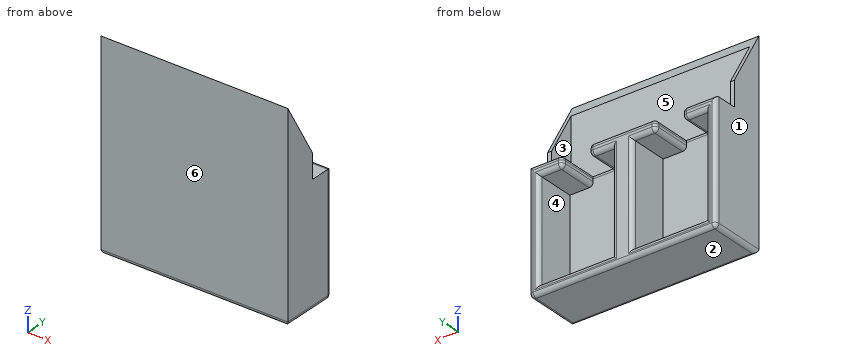
from build123d import *

# Parameters (mm, degrees)
SKETCH1_W               = 140
SKETCH1_H               = 90
BOSS_EXTRUDE1_DEPTH     = 42
CUT_EXTRUDE1_DEPTH      = 30
FILLET2_R               = 3
SKETCH3_W               = 140
SKETCH3_H               = 60
BOSS_EXTRUDE2_DEPTH     = 5
SKETCH4_W               = 3
SKETCH4_H               = 60
BOSS_EXTRUDE3_DEPTH     = 19
CUT_EXTRUDE2_DEPTH      = 172.650808329
CUT_EXTRUDE2_DEPTH_BACK = 172.650808329


with BuildPart() as part:
    # Sketch1 → Boss-Extrude1 (new body)
    with BuildSketch(Plane(origin=(0, 0, 0), x_dir=(1, 0, 0), z_dir=(0, 1, 0))):
        with Locations((70, 45)):
            Rectangle(SKETCH1_W, SKETCH1_H)
    extrude(amount=BOSS_EXTRUDE1_DEPTH)

    # Sketch2 → Cut-Extrude1 (cut)
    with BuildSketch(Plane(origin=(0, 42, 0), x_dir=(1, 0, 0), z_dir=(0, 1, 0))):
        Polygon((7.5, 8), (7.5, 83), (62.5, 83), (62.5, 8), (45, 8), (45, 0), (25, 0), (25, 8), align=None)
        Polygon((77.5, 8), (77.5, 83), (132.5, 83), (132.5, 8), (115, 8), (115, 0), (95, 0), (95, 8), align=None)
    extrude(amount=-CUT_EXTRUDE1_DEPTH, mode=Mode.SUBTRACT)

    # Fillet2
    fillet2_edges = [part.edges().sort_by_distance(p)[0] for p in [
        (140, 42, -45),
        (70, 42, 0),
        (127.5, 42, 0),
        (70, 42, -90),
        (25, 27, -8),
        (45, 27, -8),
        (35, 12, 0),
        (45, 27, 0),
        (25, 27, 0),
        (16.25, 42, -8),
        (25, 42, -4),
        (45, 42, -4),
        (53.75, 42, -8),
        (62.5, 42, -45.5),
        (35, 42, -83),
        (7.5, 42, -45.5),
        (95, 27, -8),
        (115, 27, -8),
        (105, 12, 0),
        (115, 27, 0),
        (95, 27, 0),
        (86.25, 42, -8),
        (95, 42, -4),
        (115, 42, -4),
        (123.75, 42, -8),
        (132.5, 42, -45.5),
        (105, 42, -83),
        (77.5, 42, -45.5),
        (0, 42, -45),
        (70, 0, -90),
        (0, 21, -90),
        (140, 21, -90),
        (12.5, 42, 0),
    ]]
    fillet(fillet2_edges, radius=FILLET2_R)

    # Sketch3 → Boss-Extrude2 (add)
    with BuildSketch(Plane(origin=(0, 0, 0), x_dir=(1, 0, 0), z_dir=(0, 1, 0))):
        with Locations((70, -30)):
            Rectangle(SKETCH3_W, SKETCH3_H)
    extrude(amount=BOSS_EXTRUDE2_DEPTH)

    # Sketch4 → Boss-Extrude3 (add)
    with BuildSketch(Plane(origin=(0, 5, 0), x_dir=(1, 0, 0), z_dir=(0, 1, 0))):
        with Locations((1.5, -30)):
            Rectangle(SKETCH4_W, SKETCH4_H)
        with Locations((138.5, -30)):
            Rectangle(SKETCH4_W, SKETCH4_H)
    extrude(amount=BOSS_EXTRUDE3_DEPTH)

    # Sketch5 → Cut-Extrude2 (cut, two sides: drawn at the far end of the back side and taken through both)
    with BuildSketch(Plane.ZY.offset(-CUT_EXTRUDE2_DEPTH_BACK)):
        Polygon((60, 0), (8.038475773, 30), (60, 30), align=None)
    extrude(amount=CUT_EXTRUDE2_DEPTH + CUT_EXTRUDE2_DEPTH_BACK, mode=Mode.SUBTRACT)


solid = part.part
Verification items for the finished model (mm, model axes). Face numbers are marked on the shaded views. A direction names the side the tool comes from. Coordinates: 2 decimals unless noted, no trailing zeros. Order: outer loops, then holes, each group sorted by start corner. A loop starts at its lowest first (then second) coordinate and runs counter-clockwise, first axis right, second up. Notation, with made-up numbers: M -5,8 L 17,8 A33 cw 17,39 Z; hole C 58,-11.5 d7. An arc over 180 degrees is marked long. Return JSON: item names as keys, results as strings.
1) Cross-section at C-C, the plane z = -76.5. Record the boundary of the cut face in (x, y).
Answer list:
{"outline": "M 0,0 L 140,0 L 140,39 A3 ccw 137,42 L 135.5,42 A3 ccw 132.5,39 L 132.5,12 L 77.5,12 L 77.5,39 A3 ccw 74.5,42 L 65.5,42 A3 ccw 62.5,39 L 62.5,12 L 7.5,12 L 7.5,39 A3 ccw 4.5,42 L 3,42 A3 ccw 0,39 Z"}
2) Thickness scan on L1, parallel to X at y = 31, z = -64.5; L2, parallel to Z at x = 21, y = 28.5; L3, parallel to X at y = 17, z = 9. Record the ranges inside material, lowest first. Write a range as [from, to].
Answer list:
{"L1": "[0, 7.5], [62.5, 77.5], [132.5, 140]", "L2": "[-90, -83], [-8, 0]", "L3": "[0, 3], [137, 140]"}
3) Release check for a two-part mould opening along X. For the marked faces 1, 2 and 3 record: +X half, -X half, draft (parallel to the pull), parting line (faces both ways), or undercut.
Answer list:
{"face 1": "-X half", "face 2": "draft", "face 3": "undercut"}
4) Gauge pin test, flat ends, axial feed: pin 1 (8 mm diameter, centred on x = 23, y = 20.5, fed in from +Z); pin 2 (10 mm diameter, centred on x = 112, y = 23, fed in from +Z); pin 3 (12 mm diameter, centred on x = 31.5, z = -14.5, fed in from +Y). Record the tip position at first contact, or that the pin passes through.
Answer list:
{"pin 1": "z = 0", "pin 2": "z = -0.17", "pin 3": "y = 12"}
5) Cross-section at A-A, the plane x = 39.5. Record the boundary of the cut face in (y, z), and give its area (3 significant figures).
Answer list:
{"outline": "M 0,-87 A3 ccw 3,-90 L 39,-90 A3 ccw 42,-87 L 42,-86 A3 ccw 39,-83 L 12,-83 L 12,-3 A3 ccw 9,0 L 5,0 L 5,51.34 L 0,60 Z", "area": "1,560 mm2"}
6) Access from +Z, -Z, +X, -X, +Y, -Y to the whole of each face (thin tool, end or side, straight path). Record for the marked faces 4, 5 and 6.
Answer list:
{"face 4": "+Y", "face 5": "+Z, +Y", "face 6": "+Z, -Z, +X, -X, -Y"}
7) Cross-section at D-D, the plane z = 49. Record the boundary of the cut face in (x, y), and give its area (3 significant figures).
Answer list:
{"outline": "M 0,0 L 140,0 L 140,6.35 L 137,6.35 L 137,5 L 3,5 L 3,6.35 L 0,6.35 Z", "area": "708 mm2"}
